Geometry check sheet. Reference: the model listing, model coordinates, mm. A direction names the side the tool comes from. Round coordinates to 2 decimals unless told otherwise and drop trailing zeros. Order: outer loops, then holes, each group sorted by start corner. A loop starts at its lowest first (then second) coordinate and runs counter-clockwise, first axis right, second up. Notation, with made-up numbers: (-32.5, 25) - (8.5, 25) arc R16 cw to (8.5, 47) - close; hole circle Ø6 at (77, -29.5). An arc over 180 degrees is marked (long way). Use a Markdown table: item, result. Add a question column.
(1) Gauge pin test, flat ends, axial feed: P1, Ø7, axis at x = 0, z = 15, coming from the -Y side; P2, Ø5, axis at x = 3.5, z = 14, coming from the -Y side; P3, Ø4.5, axis at x = -19.5, y = 5.5, coming from the +Z side; P4, Ø1.8, axis at y = 5, z = 18.5, coming from the -X side. Record the tip position at first contact, or that the pin passes through.
(2) Section check C-C on x = 0. Record the boundary of the cut face in (y, z).
(3) Section check A-A on y = 6.5. Record the boundary of the cut face in (x, z).
(4) Section check D-D on z = 18.5. Record the boundary of the cut face in (x, y).
(5) Section check B-B on z = 3.75. Record the boundary of the cut face in (x, y).
(6) Thickness scan on line 1 along Z through (x, y) = (0, 1.1); line 2 along X through (y, z) = (4, 1.65); line 3 along Y through (x, z) = (23.25, 3.35). Record the ranges inside material, lowest first. Write a range as [from, to].
(7) Access from +Z, -Z, +X, -X, +Y, -Y to the whole of each face (thin tool, end or side, straight path). Record for faces 4 (the face through (-18.859, 3.944, 3.797)), 5 (the face through (21.6, 4.07, 3.04)), 6 (the face through (11, 4, 18)).
(8) Mould release check, pull along Z, two halves, no side actions. Record for faces 1 (the face through (-25, 3, 0)), 2 (the face through (0, 0, 6)), 3 (the face through (1.756, 0.986, 22.907)): released by +Z, released by -Z, zero draft, split by the parting line, or undercut.
```python
from build123d import *

# Parameters (mm, degrees)
SKETCH1_W                                = 53
SKETCH1_H                                = 26
BOSS_EXTRUDE1_DEPTH                      = 8
SKETCH2_W                                = 15.5
SKETCH2_H                                = 16
CUT_EXTRUDE1_DEPTH                       = 38.976966704
SKETCH3_W                                = 15.5
SKETCH3_H                                = 16
CUT_EXTRUDE2_DEPTH                       = 38.976966704
SKETCH4_W                                = 40.000000023
SKETCH4_H                                = 5
CUT_EXTRUDE3_DEPTH                       = 38.976966704
CBORE_FOR_M10_HEX_HEAD_BOLT1_D           = 11.4
CBORE_FOR_M10_HEX_HEAD_BOLT1_CBORE_D     = 16.2
CBORE_FOR_M10_HEX_HEAD_BOLT1_CBORE_DEPTH = 2
M4X0_7_TAPPED_HOLE1_D                    = 3.3
M4X0_7_TAPPED_HOLE1_DEPTH                = 6
M4X0_7_TAPPED_HOLE1_TIP                  = 0.991420021
FILLET1_R                                = 4
FILLET2_R                                = 5


with BuildPart() as part:
    # Sketch1 → Boss-Extrude1 (new body)
    with BuildSketch(Plane.XZ):
        with Locations((0, 13)):
            Rectangle(SKETCH1_W, SKETCH1_H)
    extrude(amount=-BOSS_EXTRUDE1_DEPTH)

    # Sketch2 → Cut-Extrude1 (cut, through all)
    with BuildSketch(Plane(origin=(0, 8, 0), x_dir=(-1, 0, 0), z_dir=(0, 1, 0))):
        with Locations((-18.75, 18)):
            Rectangle(SKETCH2_W, SKETCH2_H)
    extrude(amount=-CUT_EXTRUDE1_DEPTH, mode=Mode.SUBTRACT)

    # Sketch3 → Cut-Extrude2 (cut, through all)
    with BuildSketch(Plane(origin=(0, 8, 0), x_dir=(-1, 0, 0), z_dir=(0, 1, 0))):
        with Locations((18.75, 18)):
            Rectangle(SKETCH3_W, SKETCH3_H)
    extrude(amount=-CUT_EXTRUDE2_DEPTH, mode=Mode.SUBTRACT)

    # Sketch4 → Cut-Extrude3 (cut, through all)
    with BuildSketch(Plane(origin=(0, 8, 0), x_dir=(-1, 0, 0), z_dir=(0, 1, 0))):
        with Locations((1.2e-08, 2.5)):
            Rectangle(SKETCH4_W, SKETCH4_H)
    extrude(amount=-CUT_EXTRUDE3_DEPTH, mode=Mode.SUBTRACT)

    # CBORE for M10 Hex Head Bolt1 (through all)
    with Locations(Plane(origin=(0, 0, 0), x_dir=(-1, 0, 0), z_dir=(0, -1, 0))):
        with Locations((0, -15)):
            CounterBoreHole(CBORE_FOR_M10_HEX_HEAD_BOLT1_D / 2, CBORE_FOR_M10_HEX_HEAD_BOLT1_CBORE_D / 2, CBORE_FOR_M10_HEX_HEAD_BOLT1_CBORE_DEPTH)

    # M4x0.7 Tapped Hole1
    with Locations(Plane(origin=(0, 0, 0), x_dir=(-1, 0, 0), z_dir=(0, 0, -1))):
        with Locations((-23.25, 4), (23.25, 4)):
            Hole(M4X0_7_TAPPED_HOLE1_D / 2, depth=M4X0_7_TAPPED_HOLE1_DEPTH)
            with Locations((0, 0, -(M4X0_7_TAPPED_HOLE1_DEPTH + M4X0_7_TAPPED_HOLE1_TIP / 2))):  # 118° drill point
                Cone(0, M4X0_7_TAPPED_HOLE1_D / 2, M4X0_7_TAPPED_HOLE1_TIP, mode=Mode.SUBTRACT)

    # Fillet1
    fillet1_edges = [part.edges().sort_by_distance(p)[0] for p in [
        (20, 4, 5),
        (-20.000000023, 4, 5),
    ]]
    fillet(fillet1_edges, radius=FILLET1_R)

    # Fillet2
    fillet2_edges = [part.edges().sort_by_distance(p)[0] for p in [
        (11, 4, 10),
        (26.5, 4, 10),
        (11, 4, 26),
        (-11, 4, 26),
        (-26.5, 4, 10),
        (-11, 4, 10),
    ]]
    fillet(fillet2_edges, radius=FILLET2_R)


solid = part.part
```
Check sheet entries:
| question | item | result |
|---|---|---|
| 1 | P1 | passes through |
| 1 | P2 | stops at y = 2 |
| 1 | P3 | stops at z = 10 |
| 1 | P4 | stops at x = -11 |
| 2 | outline | (0, 5) - (8, 5) - (8, 9.3) - (2, 9.3) - (2, 6.9) - (0, 6.9) - close; (0, 23.1) - (2, 23.1) - (2, 20.7) - (8, 20.7) - (8, 26) - (0, 26) - close |
| 3 | outline | (-26.5, 0) - (-20, 0) - (-20, 1) arc R4 cw to (-16, 5) - (16, 5) arc R4 cw to (20, 1) - (20, 0) - (26.5, 0) - (26.5, 5) arc R5 ccw to (21.5, 10) - (16, 10) arc R5 cw to (11, 15) - (11, 21) arc R5 ccw to (6, 26) - (-6, 26) arc R5 ccw to (-11, 21) - (-11, 15) arc R5 cw to (-16, 10) - (-21.5, 10) arc R5 ccw to (-26.5, 5) - close; hole circle Ø11.4 at (0, 15) |
| 4 | outline | (-11, 0) - (-7.3, 0) - (-7.3, 2) - (-4.5, 2) - (-4.5, 8) - (-11, 8) - close; (4.5, 2) - (7.3, 2) - (7.3, 0) - (11, 0) - (11, 8) - (4.5, 8) - close |
| 5 | outline | (-26.5, 0) - (-18.9, 0) - (-18.9, 8) - (-26.5, 8) - close; (18.9, 0) - (26.5, 0) - (26.5, 8) - (18.9, 8) - close; hole circle Ø3.3 at (-23.25, 4); hole circle Ø3.3 at (23.25, 4) |
| 6 | line 1 | z = [5, 6.9], [23.1, 26] |
| 6 | line 2 | x = [-26.5, -24.9], [-21.6, -19.95], [19.95, 21.6], [24.9, 26.5] |
| 6 | line 3 | y = [0, 2.35], [5.65, 8] |
| 7 | face 4 | -Z, +Y, -Y |
| 7 | face 5 | -Z |
| 7 | face 6 | +Z, +X, +Y, -Y |
| 8 | face 1 | released by -Z |
| 8 | face 2 | zero draft |
| 8 | face 3 | undercut |
